```python
from build123d import *

# Parameters (mm, degrees)
SKETCH1_R           = 4.7625
SKETCH1_R_2         = 3.175
BOSS_EXTRUDE1_DEPTH = 3.175
BOSS_EXTRUDE2_START = -0.79375
SKETCH2_R           = 5.3975
SKETCH2_R_2         = 4.7625
BOSS_EXTRUDE2_DEPTH = 0.79375
SKETCH3_R           = 5.000625
SKETCH3_R_2         = 3.571875
CUT_EXTRUDE1_DEPTH  = 0.0254
CUT_EXTRUDE2_START  = -0.0254
SKETCH4_R           = 4.365625
SKETCH4_R_2         = 3.571875
CUT_EXTRUDE2_DEPTH  = 0.0254


with BuildPart() as part:
    # Sketch1 → Boss-Extrude1 (new body)
    with BuildSketch(Plane.XY):
        Circle(SKETCH1_R)
        Circle(SKETCH1_R_2, mode=Mode.SUBTRACT)
    extrude(amount=BOSS_EXTRUDE1_DEPTH)

    # Sketch2 → Boss-Extrude2 (add)
    with BuildSketch(Plane.XY.offset(3.175).offset(BOSS_EXTRUDE2_START)):
        Circle(SKETCH2_R)
        Circle(SKETCH2_R_2, mode=Mode.SUBTRACT)
    extrude(amount=BOSS_EXTRUDE2_DEPTH)

    # Sketch3 → Cut-Extrude1 (cut)
    with BuildSketch(Plane.XY.offset(3.175)):
        Circle(SKETCH3_R)
        Circle(SKETCH3_R_2, mode=Mode.SUBTRACT)
    extrude(amount=-CUT_EXTRUDE1_DEPTH, mode=Mode.SUBTRACT)

    # Sketch4 → Cut-Extrude2 (cut)
    with BuildSketch(Plane(origin=(0, 0, 0), x_dir=(-1, 0, 0), z_dir=(0, 0, -1)).offset(CUT_EXTRUDE2_START)):
        Circle(SKETCH4_R)
        with Locations(Location((0, 0, 0), (0, 0, 180))):
            Circle(SKETCH4_R_2, mode=Mode.SUBTRACT)
    extrude(amount=CUT_EXTRUDE2_DEPTH, mode=Mode.SUBTRACT)


solid = part.part
```
Work out the finished part from the listing and answer in its coordinate system (mm). A direction names the side the tool comes from. Give positions to 0.01 mm unless a question says otherwise; leave off trailing zeros. Order: outer loops, then holes, each group sorted by start corner. A loop starts at its lowest first (then second) coordinate and runs counter-clockwise, first axis right, second up. Notation, with made-up numbers: (77, -22) - (83, -22) arc R8 ccw to (83, -9) - close; hole circle Ø3 at (66, 40.5). An arc over 180 degrees is marked (long way). One line per item, written item: value. Start each with the question number.
1. Each of these flat-tipped pins is pushed along its axis until it touches: pin 1 Ø4 at (x, y) = (4, -3) entering from -Z; pin 2 Ø5.5 at (x, y) = (0, 0) entering from -Z. Where does it stop, or does it pass through?
2. Consider line 1 (Y direction, x = 0, z = 2.05) (1 decimal); line 2 (X direction, y = -1.5, z = 0.5); line 3 (X direction, y = -2.75, z = 1.4). Determine where each line is inside the solid, lowest interval first.
3. Section D-D, the plane y = -4.5 is taken. Write down the section's boundary in (x, z) (3 decimals).
4. Which of the six approach directions +Z, -Z, +X, -X, +Y, -Y give full straight-line access (tool end or side, diameter ignored) to faces 5 (the face through (-0.69, -3.1, 1.57)), 6 (the face through (-3.78, -2.9, 1.17))?
5. For a pull along X with two mould halves and no side action, classify faces 1 (the face through (2.2, -3.3, 3.15)), 2 (the face through (4, 0, 0.025)), 3 (the face through (-3.978, 3.648, 2.773)), 4 (the face through (0, -5, 2.381)) as released by +X, released by -X, zero draft, split by the parting line, or undercut.
Filled sheet:
1. pin 1: z = 0
1. pin 2: through
2. line 1: -4.8 to -3.2, 3.2 to 4.8
2. line 2: -4.52 to -2.8, 2.8 to 4.52
2. line 3: -3.89 to -1.59, 1.59 to 3.89
3. outline: (-2.98, 2.381) - (-1.559, 2.381) - (-1.559, 0) - (1.559, 0) - (1.559, 2.381) - (2.98, 2.381) - (2.98, 3.175) - (2.181, 3.175) - (2.181, 3.15) - (-2.181, 3.15) - (-2.181, 3.175) - (-2.98, 3.175) - close
4. face 5: +Z, -Z
4. face 6: -Z
5. face 1: undercut
5. face 2: undercut
5. face 3: split by the parting line
5. face 4: zero draft
